Source: CAD feature listing. Evaluate the final solid. Frame: model axes, mm. A direction names the side the tool comes from. Coordinates: 2 decimals unless noted, no trailing zeros. Write each loop counter-clockwise with the first axis right and the second up, starting at its lowest first coordinate (ties: lowest second). Pieces come first, ordered by that corner, then holes. Notation, with made-up numbers: M 58.25,41.5 L 87.25,41.5 A16 ccw 87.25,60.5 Z; hole C 57,87 d3. An arc over 180 degrees is marked long. One line per item, written item: value. Start each with the question number.
Item 1: Cut plane D-D, the plane x = 94. Output: boundary loops of the cut face in (y, z).
Item 2: Mould query, pull axis Y, two halves, no side actions, for faces 1 (the flat face through (-1, 51, 8)), 2 (the flat face through (0, 51, 7)), 3 (the flat face through (51, -1, 8)). Classes: released by +Y, released by -Y, zero draft, split by the parting line, or undercut.
Item 3: Pin query (flat end, axial travel): P1, Ø2, axis at x = 32, y = 92, coming from the -Z side. Return the tip coordinate at first contact, or that it passes through.
Item 4: Ray query, L1, parallel to Y at x = 98, z = 13.5; L2, parallel to Z at x = 60, y = 9. Return the intervals inside material, ascending. Write a range as from..to.
Item 5: Cut plane B-B, the plane z = 11.5. Output: boundary loops of the cut face in (x, y).
Item 6: Set-up query: faces 4 (the flat face through (105, 51, 8)), 5 (the flat face through (104, 51, 7)). Return all of +Z, -Z, +X, -X, +Y, -Y with unobstructed straight access to the full face (end or side cutting, diameter ignored); none if empty.
Item 7: Cut plane A-A, the plane x = 81. Output: boundary loops of the cut face in (y, z), then the cut area to 3 significant figures.
```python
from build123d import *

# Parameters (mm, degrees)
SKETCH1_W           = 106
SKETCH1_H           = 106
SKETCH1_W_2         = 104
SKETCH1_H_2         = 104
BOSS_EXTRUDE1_DEPTH = 15
SKETCH2_W           = 106
SKETCH2_H           = 106
SKETCH2_W_2         = 74
SKETCH2_H_2         = 74
BOSS_EXTRUDE2_DEPTH = 1


with BuildPart() as part:
    # Sketch1 → Boss-Extrude1 (new body)
    with BuildSketch(Plane.XY):
        with Locations((52, 52)):
            Rectangle(SKETCH1_W, SKETCH1_H)
        with Locations((52, 52)):
            Rectangle(SKETCH1_W_2, SKETCH1_H_2, mode=Mode.SUBTRACT)
    extrude(amount=BOSS_EXTRUDE1_DEPTH)

    # Sketch2 → Boss-Extrude2 (add)
    with BuildSketch(Plane.XY.offset(15)):
        with Locations((52, 52)):
            Rectangle(SKETCH2_W, SKETCH2_H)
        with Locations((52, 52)):
            Rectangle(SKETCH2_W_2, SKETCH2_H_2, mode=Mode.SUBTRACT)
    extrude(amount=BOSS_EXTRUDE2_DEPTH)


solid = part.part
```
From the geometry:
1. outline: M -1,0 L 0,0 L 0,15 L 104,15 L 104,0 L 105,0 L 105,16 L -1,16 Z
2. face 1: zero draft
2. face 2: undercut
2. face 3: released by -Y
3. P1: stops at z = 15
4. L1: y = -1..0, 104..105
4. L2: z = 15..16
5. outline: M -1,-1 L 105,-1 L 105,105 L -1,105 Z; hole M 0,0 L 104,0 L 104,104 L 0,104 Z
6. face 4: +Z, -Z, +X, +Y, -Y
6. face 5: -Z
7. outline: M -1,0 L 0,0 L 0,15 L 15,15 L 15,16 L -1,16 Z; M 89,15 L 104,15 L 104,0 L 105,0 L 105,16 L 89,16 Z
7. area: 62.0 mm²
